```python
from build123d import *

# Parameters (mm, degrees)
SKETCH1_R           = 9
SKETCH1_R_2         = 59.5
BOSS_EXTRUDE1_DEPTH = 0.5


with BuildPart() as part:
    # Sketch1 → Boss-Extrude1 (new body)
    with BuildSketch(Plane.XY):
        with BuildLine():
            Line((-53, 84), (53, 84))
            ThreePointArc((53, 84), (69.970562748, 76.970562748), (77, 60))
            Line((77, 60), (77, -60))
            ThreePointArc((77, -60), (69.970562748, -76.970562748), (53, -84))
            Line((53, -84), (-53, -84))
            ThreePointArc((-53, -84), (-69.970562748, -76.970562748), (-77, -60))
            Line((-77, -60), (-77, 60))
            ThreePointArc((-77, 60), (-69.970562748, 76.970562748), (-53, 84))
        make_face()
        with Locations((53, 60)):
            Circle(SKETCH1_R, mode=Mode.SUBTRACT)
        with Locations(Location((-53, 60, 0), (0, 0, 180))):
            Circle(SKETCH1_R, mode=Mode.SUBTRACT)
        with Locations(Location((53, -60, 0), (0, 0, 180))):
            Circle(SKETCH1_R, mode=Mode.SUBTRACT)
        with Locations((-53, -60)):
            Circle(SKETCH1_R, mode=Mode.SUBTRACT)
        Circle(SKETCH1_R_2, mode=Mode.SUBTRACT)
    extrude(amount=BOSS_EXTRUDE1_DEPTH)


solid = part.part
```
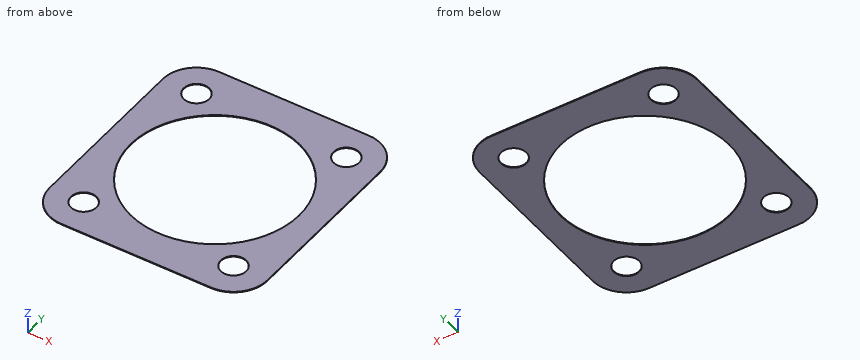
Geometry: final body of the model. Coordinates: model frame, mm. Coordinates: 2 decimals unless noted, no trailing zeros. Order: outer loops, then holes, each group sorted by start corner. A loop starts at its lowest first (then second) coordinate and runs counter-clockwise, first axis right, second up. Notation, with made-up numbers: (-25, -20) - (6, -20) arc R26 cw to (6, 17) - close; hole circle Ø11 at (63, 11.5). An arc over 180 degrees is marked (long way). Write each question's results on one line, items separated by ' | '.
1) Section C-C, the plane z = 0.1. Return loops of the section in (x, y), plus the area to 3 significant figures.
Results list:
outline: (-77, -60) arc R24 ccw to (-53, -84) - (53, -84) arc R24 ccw to (77, -60) - (77, 60) arc R24 ccw to (53, 84) - (-53, 84) arc R24 ccw to (-77, 60) - close; hole circle Ø18 at (-53, -60); hole circle Ø18 at (-53, 60); hole circle Ø119 at (0, 0); hole circle Ø18 at (53, -60); hole circle Ø18 at (53, 60) | area: 13,200 mm^2
2) Line query: line 1 (Y direction, x = 0, z = 0.2); line 2 (Y direction, x = 50.5, z = 0.2); line 3 (X direction, y = 52, z = 0.45). Output: solid intervals per line, ascending. Write a range as from..to.
Results list:
line 1: -84..-59.5, 59.5..84 | line 2: -84..-68.65, -51.35..-31.46, 31.46..51.35, 68.65..84 | line 3: -77..-57.12, -48.88..-28.92, 28.92..48.88, 57.12..77
3) Section B-B, the plane x = 0. Return loops of the section in (y, z), plus the area to 3 significant figures.
Results list:
outline: (-84, 0) - (-59.5, 0) - (-59.5, 0.5) - (-84, 0.5) - close; (59.5, 0) - (84, 0) - (84, 0.5) - (59.5, 0.5) - close | area: 24.5 mm^2
4) Pin query (flat end, axial travel): pin 1 (16 mm diameter, centred on x = -53, y = -60, fed in from -Z). Return the tip coordinate at first contact, or that it passes through.
Results list:
pin 1: through
5) Section D-D, the plane x = -66. Return loops of the section in (y, z), plus the area to 3 significant figures.
Results list:
outline: (-80.17, 0) - (80.17, 0) - (80.17, 0.5) - (-80.17, 0.5) - close | area: 80.2 mm^2
6) Section A-A, the plane y = 0. Return loops of the section in (x, z), plus the area to 3 significant figures.
Results list:
outline: (-77, 0) - (-59.5, 0) - (-59.5, 0.5) - (-77, 0.5) - close; (59.5, 0) - (77, 0) - (77, 0.5) - (59.5, 0.5) - close | area: 17.5 mm^2
